```python
from build123d import *

# Parameters (mm, degrees)
SKETCH1_W                 = 57
SKETCH1_H                 = 33
BOSS_EXTRUDE1_DEPTH       = 10
SKETCH3_R                 = 3.35
CUT_EXTRUDE1_DEPTH        = 11
SKETCH4_R                 = 3.35
CUT_EXTRUDE2_DEPTH        = 11
SKETCH10_R                = 3.35
CUT_EXTRUDE5_DEPTH        = 11
SKETCH12_R                = 3.35
CUT_EXTRUDE6_DEPTH        = 11
F_8_32_TAPPED_HOLE1_D     = 3.4544
F_8_32_TAPPED_HOLE1_DEPTH = 5
F_8_32_TAPPED_HOLE1_TIP   = 1.037806461
F_0_535_40_TAPPED_HOLE1_D = 12.7


with BuildPart() as part:
    # Sketch1 → Boss-Extrude1 (new body)
    with BuildSketch(Plane(origin=(0, 0, 0), x_dir=(1, 0, 0), z_dir=(0, 1, 0))):
        with Locations((28.5, 16.5)):
            Rectangle(SKETCH1_W, SKETCH1_H)
    extrude(amount=BOSS_EXTRUDE1_DEPTH)

    # Sketch3 → Cut-Extrude1 (cut, through all)
    with BuildSketch(Plane.XZ):
        with Locations((6, -6.5)):
            Circle(SKETCH3_R)
    extrude(amount=-CUT_EXTRUDE1_DEPTH, mode=Mode.SUBTRACT)

    # Sketch4 → Cut-Extrude2 (cut, through all)
    with BuildSketch(Plane.XZ):
        with Locations((51, -26.5)):
            Circle(SKETCH4_R)
    extrude(amount=-CUT_EXTRUDE2_DEPTH, mode=Mode.SUBTRACT)

    # Sketch10 → Cut-Extrude5 (cut, through all)
    with BuildSketch(Plane.XZ):
        with Locations((6, -26.5)):
            Circle(SKETCH10_R)
    extrude(amount=-CUT_EXTRUDE5_DEPTH, mode=Mode.SUBTRACT)

    # Sketch12 → Cut-Extrude6 (cut, through all)
    with BuildSketch(Plane.XZ):
        with Locations((51, -6.5)):
            Circle(SKETCH12_R)
    extrude(amount=-CUT_EXTRUDE6_DEPTH, mode=Mode.SUBTRACT)

    # #8-32 Tapped Hole1
    with Locations(Plane(origin=(0, 0, -33), x_dir=(-1, 0, 0), z_dir=(0, 0, -1))):
        with Locations((-28.5, 5)):
            Hole(F_8_32_TAPPED_HOLE1_D / 2, depth=F_8_32_TAPPED_HOLE1_DEPTH)
            with Locations((0, 0, -(F_8_32_TAPPED_HOLE1_DEPTH + F_8_32_TAPPED_HOLE1_TIP / 2))):  # 118° drill point
                Cone(0, F_8_32_TAPPED_HOLE1_D / 2, F_8_32_TAPPED_HOLE1_TIP, mode=Mode.SUBTRACT)

    # 0.535-40 Tapped Hole1 (through all)
    with Locations(Plane(origin=(0, 10, 0), x_dir=(1, 0, 0), z_dir=(0, 1, 0))):
        with Locations((28.5, 16.5)):
            Hole(F_0_535_40_TAPPED_HOLE1_D / 2)


solid = part.part
```
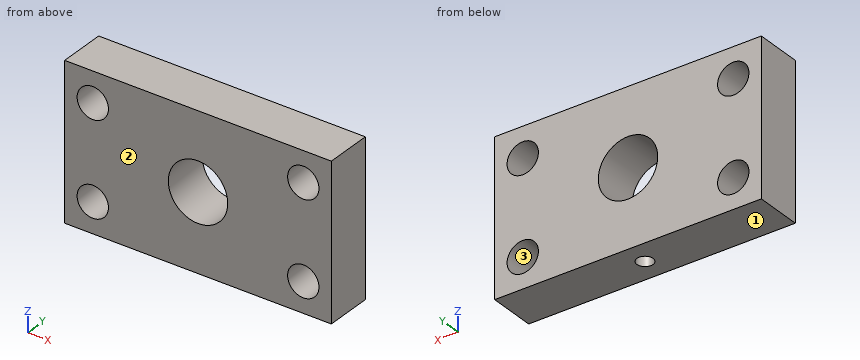
Build history of the part. All positions in model axes, mm. Face numbers are marked on the shaded views. Coordinates: 2 decimals unless noted, no trailing zeros. Write each loop counter-clockwise with the first axis right and the second up, starting at its lowest first coordinate (ties: lowest second). Pieces come first, ordered by that corner, then holes.
1. Pull direction Z, two halves, no side cores. Call the marked faces 1, 2 and 3: released by +Z, released by -Z, zero draft, split by the parting line, or undercut.
Answer block:
face 1: released by -Z
face 2: zero draft
face 3: undercut
2. Band-saw the part on C-C, the plane y = 2. Give the cut face in (x, z), and give its area (3 significant figures).
Answer block:
outline: (0, -33) - (57, -33) - (57, 0) - (0, 0) - close; hole circle Ø6.7 at (6, -26.5); hole circle Ø6.7 at (6, -6.5); hole circle Ø12.7 at (28.5, -16.5); hole circle Ø6.7 at (51, -26.5); hole circle Ø6.7 at (51, -6.5)
area: 1,610 mm2
3. Drop a flat-ended pin along its axis: pin 1 (11.5 mm diameter, centred on x = 28.5, z = -16.5, fed in from +Y). Give the stop position or say it passes through.
Answer block:
pin 1: passes through
4. Band-saw the part on D-D, the plane z = -6.5. Give the cut face in (x, y), and give its area (3 significant figures).
Answer block:
outline: (0, 0) - (2.65, 0) - (2.65, 10) - (0, 10) - close; (9.35, 0) - (47.65, 0) - (47.65, 10) - (9.35, 10) - close; (54.35, 0) - (57, 0) - (57, 10) - (54.35, 10) - close
area: 436 mm2
5. Band-saw the part on B-B, the plane x = 51. Give the cut face in (y, z).
Answer block:
outline: (0, -33) - (10, -33) - (10, -29.85) - (0, -29.85) - close; (0, -23.15) - (10, -23.15) - (10, -9.85) - (0, -9.85) - close; (0, -3.15) - (10, -3.15) - (10, 0) - (0, 0) - close
6. Drill centre lines: probe 1 along Z at (x, y) = (51, 6.75); probe 2 along X at (y, z) = (5.5, -25); probe 3 along X at (y, z) = (0.5, -27.5). Where is each one in solid material? Low to high.
Answer block:
probe 1: z = -33 to -29.85, -23.15 to -9.85, -3.15 to 0
probe 2: x = 0 to 3, 9 to 48, 54 to 57
probe 3: x = 0 to 2.8, 9.2 to 47.8, 54.2 to 57
7. Band-saw the part on A-A, the plane z = -16.5. Give the cut face in (x, y).
Answer block:
outline: (0, 0) - (22.15, 0) - (22.15, 10) - (0, 10) - close; (34.85, 0) - (57, 0) - (57, 10) - (34.85, 10) - close
